Here's how the part is built. I have some questions about the finished solid (model axes, mm). Round coordinates to 2 decimals unless told otherwise and drop trailing zeros. Order: outer loops, then holes, each group sorted by start corner. A loop starts at its lowest first (then second) coordinate and runs counter-clockwise, first axis right, second up.
```python
from build123d import *

# Parameters (mm, degrees)
SKETCH002_R  = 50
PAD002_DEPTH = 20
FILLET003_R  = 3
FILLET004_R  = 3


with BuildPart() as part:
    # Sketch002 → Pad002 (new body)
    with BuildSketch(Plane(origin=(-110, 0, 0), x_dir=(0, 0, -1), z_dir=(1, 0, 0))):
        with Locations((0.73979, -0.924742)):
            Circle(SKETCH002_R)
    extrude(amount=PAD002_DEPTH)

    # Fillet003
    fillet003_edges = [part.edges().sort_by_distance(p)[0] for p in [
        (-90, -0.924742, 49.26021),
    ]]
    fillet(fillet003_edges, radius=FILLET003_R)

    # Fillet004
    fillet004_edges = [part.edges().sort_by_distance(p)[0] for p in [
        (-110, -0.924742, 49.26021),
    ]]
    fillet(fillet004_edges, radius=FILLET004_R)


solid = part.part
```
1. I need wall thicknesses on probe 1 along Z at (x, y) = (-96.5, -18); probe 2 along Z at (x, y) = (-106, -11); probe 3 along Y at (x, z) = (-97.5, -20.5). Which ranges of each line are inside material? Lowest first, please.
Evaluation:
probe 1: z = -47.73 to 46.25
probe 2: z = -49.71 to 48.23
probe 3: y = -46.85 to 45
2. I'm going to push flat-ended pins straight in: P1, Ø1.5, axis at x = -100.5, y = 3, coming from the -Z side; P2, Ø12, axis at x = -100, z = -37.5, coming from the +Y side; P3, Ø5, axis at y = 37.5, z = -35, coming from the -X side. Where does each tip first touch, or does it pass through?
Evaluation:
P1: stops at z = -50.64
P2: stops at y = 38.49
P3: stops at x = -109.25
3. If we section it at B-B, the plane x = -108.5: Write out the boundary of the cut face in (y, z), and give its area (3 significant figures).
Evaluation:
outline: circle Ø99.2 at (-0.92, -0.74)
area: 7,730 mm2
4. If we section it at A-A, the plane x = -91.75: Write out the boundary of the cut face in (y, z).
Evaluation:
outline: circle Ø99.45 at (-0.92, -0.74)
